Geometry: final body of the model. Coordinates: model frame, mm. Give positions to 0.01 mm unless a question says otherwise; leave off trailing zeros. Loops run counter-clockwise (first coordinate to the right, second up) from the corner with the lowest first, then second, coordinate; pieces in that order, holes last. Notation, with made-up numbers: (52.25, -31) -> (74.25, -31) arc R28 cw to (74.25, -2) -> close; hole circle Ø11 at (73, 89). An arc over 180 degrees is marked (long way). One line per question, with ' | ' between items. Start each with the question number.
Item 1: Material intervals for line 1 along Z through (x, y) = (0, 0.2); line 2 along Z through (x, y) = (0, 0.75); line 3 along X through (y, z) = (0.15, -116), sorted ascending. Write a range as [from, to].
Item 2: Pin query (flat end, axial travel): P1, Ø9.5, axis at x = 0, z = 116, coming from the +Y side; P2, Ø1.8, axis at x = 0, z = 55, coming from the +Y side; P3, Ø7, axis at x = 0, z = -116, coming from the +Y side. Return the tip coordinate at first contact, or that it passes through.
Item 3: Section A-A on y = 2.6. Return loops of the section in (x, z), then the cut area to 3 significant figures.
Item 4: Section B-B on z = -116. Return loops of the section in (x, y), then the cut area to 3 significant figures.
Item 5: Mould query, pull axis Z, two halves, no side actions, for faces 1 (the flat face through (0, 0, -2)), 2 (the cylindrical face through (-0.391, 0.253, -118.974)), 3 (the cylindrical face through (-0.391, 0.253, 113.026)). Classes: released by +Z, released by -Z, zero draft, split by the parting line, or undercut.
from build123d import *

# Parameters (mm, degrees)
SKETCH1_W           = 30
SKETCH1_H           = 252
BOSS_EXTRUDE1_DEPTH = 3.5
SKETCH2_R           = 1.5
SKETCH2_R_2         = 3
CUT_EXTRUDE1_DEPTH  = 3.5
CHAMFER1_SIZE       = 3


with BuildPart() as part:
    # Sketch1 → Boss-Extrude1 (new body)
    with BuildSketch(Plane(origin=(0, 0, 0), x_dir=(1, 0, 0), z_dir=(0, 1, 0))):
        Rectangle(SKETCH1_W, SKETCH1_H)
    extrude(amount=BOSS_EXTRUDE1_DEPTH)

    # Sketch2 → Cut-Extrude1 (cut)
    with BuildSketch(Plane(origin=(0, 3.5, 0), x_dir=(1, 0, 0), z_dir=(0, 1, 0))):
        with Locations((0, 55)):
            Circle(SKETCH2_R)
        with Locations((0, -55)):
            Circle(SKETCH2_R)
        with Locations((0, 116)):
            Circle(SKETCH2_R_2)
        with Locations((0, -116)):
            Circle(SKETCH2_R_2)
    extrude(amount=-CUT_EXTRUDE1_DEPTH, mode=Mode.SUBTRACT)

    # Chamfer1
    chamfer1_edges = [part.edges().sort_by_distance(p)[0] for p in [
        (-3, 3.5, 116),
        (-3, 3.5, -116),
    ]]
    chamfer(chamfer1_edges, length=CHAMFER1_SIZE)


solid = part.part
Result sheet:
1) line 1: z = [-126, -119], [-113, -56.5], [-53.5, 53.5], [56.5, 113], [119, 126] | line 2: z = [-126, -119.25], [-112.75, -56.5], [-53.5, 53.5], [56.5, 112.75], [119.25, 126] | line 3: x = [-15, -3], [3, 15]
2) P1: stops at y = 2.25 | P2: passes through | P3: stops at y = 1
3) outline: (-15, -126) -> (15, -126) -> (15, 126) -> (-15, 126) -> close; hole circle Ø10.2 at (0, -116); hole circle Ø10.2 at (0, 116); hole circle Ø3 at (0, -55); hole circle Ø3 at (0, 55) | area: 7,380 mm²
4) outline: (-15, 0) -> (-3, 0) -> (-3, 0.5) -> (-6, 3.5) -> (-15, 3.5) -> close; (3, 0) -> (15, 0) -> (15, 3.5) -> (6, 3.5) -> (3, 0.5) -> close | area: 75.0 mm²
5) face 1: zero draft | face 2: undercut | face 3: undercut
